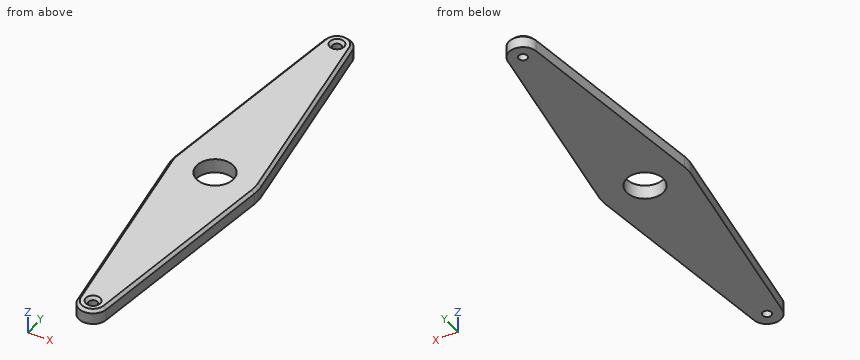
from build123d import *

# Parameters (mm, degrees)
BOSS_EXTRUDE1_DEPTH      = 5
CHAMFER1_SIZE            = 1
SKETCH6_R                = 1.55
CUT_EXTRUDE2_DEPTH       = 5
CHAMFER3_SIZE            = 1
CHAMFER3_OF_MIRROR2_SIZE = 1
CUT_EXTRUDE3_REACH       = 7
SKETCH10_R               = 6.5


with BuildPart() as part:
    # Sketch1 → Boss-Extrude1 (new body)
    with BuildSketch(Plane.XY):
        with BuildLine():
            ThreePointArc((100, 68), (99.964606776, 69.029827187), (99.858594129, 70.054794521))
            Line((99.858594129, 70.054794521), (89.95286471, 141.684931507))
            ThreePointArc((89.95286471, 141.684931507), (85, 146), (80.04713529, 141.684931507))
            Line((80.04713529, 141.684931507), (70.141405871, 70.054794521))
            ThreePointArc((70.141405871, 70.054794521), (70, 68), (70.141405871, 65.945205479))
            Line((70.141405871, 65.945205479), (80.04713529, -5.684931507))
            ThreePointArc((80.04713529, -5.684931507), (85, -10), (89.95286471, -5.684931507))
            Line((89.95286471, -5.684931507), (99.858594129, 65.945205479))
            ThreePointArc((99.858594129, 65.945205479), (99.964606776, 66.970172813), (100, 68))
        make_face()
    extrude(amount=BOSS_EXTRUDE1_DEPTH)

    # Chamfer1
    chamfer1_edges = [part.edges().sort_by_distance(p)[0] for p in [
        (100, 68, 5),
        (94.905729419, 105.869863014, 5),
        (85, 146, 5),
        (75.094270581, 105.869863014, 5),
        (70, 68, 5),
        (75.094270581, 30.130136986, 5),
        (85, -10, 5),
        (94.905729419, 30.130136986, 5),
    ]]
    chamfer(chamfer1_edges, length=CHAMFER1_SIZE)

    # Sketch6 → Cut-Extrude2 (cut)
    with BuildSketch(Plane.XY.offset(5)):
        with Locations((85, 141)):
            Circle(SKETCH6_R)
    cut_extrude2 = extrude(amount=-CUT_EXTRUDE2_DEPTH, mode=Mode.SUBTRACT)

    # Chamfer3
    chamfer3_edges = [part.edges().sort_by_distance(p)[0] for p in [
        (83.45, 141, 5),
    ]]
    chamfer(chamfer3_edges, length=CHAMFER3_SIZE)

    # Mirror2: Cut-Extrude2 across plane
    add(cut_extrude2.mirror(Plane(origin=(0, 68, 0), x_dir=(0, 0, 1), z_dir=(0, -1, 0))), mode=Mode.SUBTRACT)

    # Chamfer3 of Mirror2
    chamfer3_of_mirror2_edges = [part.edges().sort_by_distance(p)[0] for p in [
        (83.45, -5, 5),
    ]]
    chamfer(chamfer3_of_mirror2_edges, length=CHAMFER3_OF_MIRROR2_SIZE)

    # Sketch10 → Cut-Extrude3 (cut, up to next)
    with BuildSketch(Plane(origin=(0, 0, 0), x_dir=(-1, 0, 0), z_dir=(0, 0, -1)), mode=Mode.PRIVATE) as cut_extrude3_sk1:
        with Locations((-85, 68)):
            Circle(SKETCH10_R)
    cut_extrude3_tool1 = extrude(cut_extrude3_sk1.sketch, amount=-CUT_EXTRUDE3_REACH, mode=Mode.PRIVATE) & part.part
    add(cut_extrude3_tool1.solids().sort_by_distance((85, 68, 0))[0], mode=Mode.SUBTRACT)


solid = part.part
Work out the finished part from the listing and answer in its coordinate system (mm). Give positions to 0.01 mm unless a question says otherwise; leave off trailing zeros. Loops run counter-clockwise (first coordinate to the right, second up) from the corner with the lowest first, then second, coordinate; pieces in that order, holes last. Notation, with made-up numbers: (10.25, 26.5) - (41.25, 26.5) arc R14 cw to (41.25, 34.5) - close; hole circle Ø1 at (25.5, -28.5). An arc over 180 degrees is marked (long way). Answer in a Markdown table with one row per item.
(1) Section A-A (x = 85) is taken. Give the vertices of the cut face in (y, z).
Results list:
| item | result |
|---|---|
| outline | (-10, 0) - (-6.55, 0) - (-6.55, 4) - (-7.55, 5) - (-9, 5) - (-10, 4) - close; (-3.45, 0) - (61.5, 0) - (61.5, 5) - (-2.45, 5) - (-3.45, 4) - close; (74.5, 0) - (139.45, 0) - (139.45, 4) - (138.45, 5) - (74.5, 5) - close; (142.55, 0) - (146, 0) - (146, 4) - (145, 5) - (143.55, 5) - (142.55, 4) - close |
(2) Flat-ended cylindrical pins translate along their axes: pin 1 Ø1.5 at (y, z) = (39, 3) entering from +X; pin 2 Ø3 at (x, y) = (94.5, 66) entering from -Z; pin 3 Ø1.5 at (y, z) = (89, 1) entering from +X; pin 4 Ø5 at (x, y) = (85, -5) entering from +Z. Find the tip coordinate at first contact, or state that the pin passes through.
Results list:
| item | result |
|---|---|
| pin 1 | stops at x = 96.24 |
| pin 2 | stops at z = 0 |
| pin 3 | stops at x = 97.34 |
| pin 4 | stops at z = 4.95 |
(3) Section D-D (x = 76.75) is taken. Give the vertices of the cut face in (y, z), and give its area (3 significant figures).
Results list:
| item | result |
|---|---|
| outline | (18.16, 0) - (117.84, 0) - (117.84, 4) - (110.54, 5) - (25.46, 5) - (18.16, 4) - close |
| area | 491 mm² |
(4) Section C-C (y = 113.5) is taken. Give the vertices of the cut face in (x, z), and give its area (3 significant figures).
Results list:
| item | result |
|---|---|
| outline | (76.15, 0) - (93.85, 0) - (93.85, 4) - (92.84, 5) - (77.16, 5) - (76.15, 4) - close |
| area | 87.5 mm² |
(5) Section B-B (z = 1.5) is taken. Give the vertices of the cut face in (x, y), and give its area (3 significant figures).
Results list:
| item | result |
|---|---|
| outline | (70.14, 65.95) - (80.05, -5.68) arc R5 ccw to (89.95, -5.68) - (99.86, 65.95) arc R15 ccw to (99.86, 70.05) - (89.95, 141.68) arc R5 ccw to (80.05, 141.68) - (70.14, 70.05) arc R15 ccw to start; hole circle Ø13 at (85, 68); hole circle Ø3.1 at (85, -5); hole circle Ø3.1 at (85, 141) |
| area | 2,880 mm² |
(6) Consider L1, parallel to Y at x = 85, z = 1.05; L2, parallel to X at y = 67.5, z = 1.6; L3, parallel to Y at x = 87.5, z = 0.7. Determine where each line is inside the solid, lowest interval first. Write a range as [from, to].
Results list:
| item | result |
|---|---|
| L1 | y = [-10, -6.55], [-3.45, 61.5], [74.5, 139.45], [142.55, 146] |
| L2 | x = [70.01, 78.52], [91.48, 99.99] |
| L3 | y = [-9.33, 62], [74, 145.33] |
